```python
from build123d import *

# Parameters (mm, degrees)
SALIENTE_EXTRUIR1_DEPTH  = 2
CROQUIS2_W               = 30
CROQUIS2_H               = 17
CORTAR_EXTRUIR1_DEPTH    = 8
CROQUIS4_W               = 63.5
CROQUIS4_H               = 4
SALIENTE_EXTRUIR2_DEPTH  = 48.5
CROQUIS5_W               = 43.5
CROQUIS5_H               = 2.5
SALIENTE_EXTRUIR3_DEPTH  = 35
CROQUIS7_R               = 1.5
CORTAR_EXTRUIR2_DEPTH    = 9
CROQUIS8_R               = 1.5
CORTAR_EXTRUIR3_DEPTH    = 23
SALIENTE_EXTRUIR4_DEPTH  = 2
CROQUIS13_R              = 1.5
CORTAR_EXTRUIR4_DEPTH    = 2
CROQUIS16_W              = 3
CROQUIS16_H              = 31
SALIENTE_EXTRUIR7_DEPTH  = 2
CROQUIS17_W              = 15
CROQUIS17_H              = 3
SALIENTE_EXTRUIR8_DEPTH  = 25
CROQUIS21_W              = 15
CROQUIS21_H              = 3
SALIENTE_EXTRUIR9_DEPTH  = 2
CROQUIS25_R              = 3.826074219
CORTAR_EXTRUIR6_DEPTH    = 2
CROQUIS28_W              = 44.201296129
CROQUIS28_H              = 11.418561917
SALIENTE_EXTRUIR10_DEPTH = 2
CROQUIS30_W              = 15
CROQUIS30_H              = 3
SALIENTE_EXTRUIR11_DEPTH = 8
CROQUIS31_W              = 14
CROQUIS31_H              = 9
CORTAR_EXTRUIR7_DEPTH    = 2
CROQUIS33_W              = 39.5
CROQUIS33_H              = 1
SALIENTE_EXTRUIR13_DEPTH = 2
CROQUIS36_W              = 4.944902354
CROQUIS36_H              = 4.974433571
CROQUIS36_R              = 1.566702584
SALIENTE_EXTRUIR14_DEPTH = 2
CROQUIS37_R              = 2.242266835
CORTAR_EXTRUIR8_DEPTH    = 2
CROQUIS38_W              = 1.939564783
CROQUIS38_H              = 6.647351579
SALIENTE_EXTRUIR18_DEPTH = 2
CROQUIS39_R              = 2.608387943
CORTAR_EXTRUIR9_DEPTH    = 2
CROQUIS40_R              = 2.045540146
CORTAR_EXTRUIR10_DEPTH   = 2
CROQUIS41_R              = 2.280483158
CORTAR_EXTRUIR11_DEPTH   = 2
CROQUIS42_W              = 15
CROQUIS42_H              = 25
SALIENTE_EXTRUIR19_DEPTH = 5
CROQUIS43_R              = 1.6
CORTAR_EXTRUIR12_DEPTH   = 10


with BuildPart() as part:
    # Croquis1 → Saliente-Extruir1 (new body)
    with BuildSketch(Plane(origin=(0, 0, 0), x_dir=(1, 0, 0), z_dir=(0, 1, 0))):
        Polygon((25, 42), (-25, 42), (-25, -29), (-50, -29), (-50, -42), (50, -42), (50, -29), (25, -29), align=None)
    extrude(amount=SALIENTE_EXTRUIR1_DEPTH)

    # Croquis2 → Cortar-Extruir1 (cut)
    with BuildSketch(Plane(origin=(0, 0, 0), x_dir=(1, 0, 0), z_dir=(0, 1, 0))):
        with Locations((0, 33.5)):
            Rectangle(CROQUIS2_W, CROQUIS2_H)
    extrude(amount=CORTAR_EXTRUIR1_DEPTH, mode=Mode.SUBTRACT)

    # Croquis4 → Saliente-Extruir2 (add)
    with BuildSketch(Plane(origin=(0, 0, 0), x_dir=(1, 0, 0), z_dir=(0, 1, 0))):
        with Locations((0, -40)):
            Rectangle(CROQUIS4_W, CROQUIS4_H)
    extrude(amount=SALIENTE_EXTRUIR2_DEPTH)

    # Croquis5 → Saliente-Extruir3 (add)
    with BuildSketch(Plane(origin=(0, 0, 0), x_dir=(1, 0, 0), z_dir=(0, 1, 0))):
        with Locations((0, -3.75)):
            Rectangle(CROQUIS5_W, CROQUIS5_H)
    extrude(amount=SALIENTE_EXTRUIR3_DEPTH)

    # Croquis7 → Cortar-Extruir2 (cut, symmetric)
    with BuildSketch(Plane(origin=(0, 0, 38), x_dir=(-1, 0, 0), z_dir=(0, 0, -1))):
        with Locations(Location((-18, 43.25, 0), (0, 0, 180))):
            Circle(CROQUIS7_R)
        with Locations(Location((18, 43.25, 0), (0, 0, 180))):
            Circle(CROQUIS7_R)
        with Locations(Location((18, 7.25, 0), (0, 0, 180))):
            Circle(CROQUIS7_R)
        with Locations(Location((-18, 7.25, 0), (0, 0, 180))):
            Circle(CROQUIS7_R)
    extrude(amount=CORTAR_EXTRUIR2_DEPTH, both=True, mode=Mode.SUBTRACT)

    # Croquis8 → Cortar-Extruir3 (cut)
    with BuildSketch(Plane(origin=(0, 0, 2.5), x_dir=(-1, 0, 0), z_dir=(0, 0, -1))):
        with Locations((-15, 27.5)):
            Circle(CROQUIS8_R)
        with Locations((15, 9.5)):
            Circle(CROQUIS8_R)
        with Locations((15, 27.5)):
            Circle(CROQUIS8_R)
        with Locations((-15, 9.5)):
            Circle(CROQUIS8_R)
    extrude(amount=-CORTAR_EXTRUIR3_DEPTH, mode=Mode.SUBTRACT)



with BuildPart() as body_2:
    # Croquis12 → Saliente-Extruir4 (new body)
    with BuildSketch(Plane(origin=(0, 35, -35), x_dir=(1, 0, 0), z_dir=(0, -1, 0))):
        Polygon((21.25, 44.75), (-21.25, 44.75), (-21.25, 54.25), (-30.25, 54.25), (-30.25, 23.25), (-21.25, 23.25), (-21.25, 32.75), (21.25, 32.75), (21.25, 23.25), (30.25, 23.25), (30.25, 54.25), (21.25, 54.25), align=None)
    extrude(amount=-SALIENTE_EXTRUIR4_DEPTH)

    # Croquis13 → Cortar-Extruir4 (cut)
    with BuildSketch(Plane(origin=(0, 37, 0), x_dir=(1, 0, 0), z_dir=(0, 1, 0))):
        with Locations(Location((23, -15.25, 0), (0, 0, 270))):
            Circle(CROQUIS13_R)
        with Locations(Location((23, 7.75, 0), (0, 0, 90))):
            Circle(CROQUIS13_R)
        with Locations(Location((-23, 7.75, 0), (0, 0, 270))):
            Circle(CROQUIS13_R)
        with Locations(Location((-23, -15.25, 0), (0, 0, 90))):
            Circle(CROQUIS13_R)
    extrude(amount=-CORTAR_EXTRUIR4_DEPTH, mode=Mode.SUBTRACT)


with BuildPart() as part_1:
    add(part.part)

    add(body_2.part)  # Saliente-Extruir7 merges body 2
    # Croquis16 → Saliente-Extruir7 (add)
    with BuildSketch(Plane(origin=(0, 37, 0), x_dir=(1, 0, 0), z_dir=(0, 1, 0))):
        with Locations((-19.75, -3.75)):
            Rectangle(CROQUIS16_W, CROQUIS16_H)
    extrude(amount=-SALIENTE_EXTRUIR7_DEPTH)

    # Croquis17 → Saliente-Extruir8 (add)
    with BuildSketch(Plane(origin=(0, 2, 0), x_dir=(1, 0, 0), z_dir=(0, 1, 0))):
        with Locations((-0.769919921, 23.5)):
            Rectangle(CROQUIS17_W, CROQUIS17_H)
    extrude(amount=SALIENTE_EXTRUIR8_DEPTH)

    # Croquis21 → Saliente-Extruir9 (add)
    with BuildSketch(Plane(origin=(0, 27, 0), x_dir=(1, 0, 0), z_dir=(0, 1, 0))):
        with Locations((-0.769919921, 23.5)):
            Rectangle(CROQUIS21_W, CROQUIS21_H)
    extrude(amount=SALIENTE_EXTRUIR9_DEPTH)

    # Croquis25 → Cortar-Extruir6 (cut)
    with BuildSketch(Plane(origin=(0, 0, -25), x_dir=(-1, 0, 0), z_dir=(0, 0, -1))):
        with Locations((1.065680286, 20.360266958)):
            Circle(CROQUIS25_R)
    extrude(amount=-CORTAR_EXTRUIR6_DEPTH, mode=Mode.SUBTRACT)

    # Croquis28 → Saliente-Extruir10 (add)
    with BuildSketch(Plane(origin=(0, 37, 0), x_dir=(1, 0, 0), z_dir=(0, 1, 0))):
        with Locations((0.855508958, 17.459280959)):
            Rectangle(CROQUIS28_W, CROQUIS28_H)
    extrude(amount=-SALIENTE_EXTRUIR10_DEPTH)

    # Croquis30 → Saliente-Extruir11 (add)
    with BuildSketch(Plane(origin=(0, 37, 0), x_dir=(1, 0, 0), z_dir=(0, 1, 0))):
        with Locations((-0.769919921, 23.5)):
            Rectangle(CROQUIS30_W, CROQUIS30_H)
    extrude(amount=-SALIENTE_EXTRUIR11_DEPTH)

    # Croquis31 → Cortar-Extruir7 (cut)
    with BuildSketch(Plane(origin=(0, 37, 0), x_dir=(1, 0, 0), z_dir=(0, 1, 0))):
        with Locations((-1.129241311, 17.391372283)):
            Rectangle(CROQUIS31_W, CROQUIS31_H)
    extrude(amount=-CORTAR_EXTRUIR7_DEPTH, mode=Mode.SUBTRACT)

    # Croquis33 → Saliente-Extruir13 (add)
    with BuildSketch(Plane(origin=(0, 37, 0), x_dir=(1, 0, 0), z_dir=(0, 1, 0))):
        with Locations((1.5, 11.25)):
            Rectangle(CROQUIS33_W, CROQUIS33_H)
    extrude(amount=-SALIENTE_EXTRUIR13_DEPTH)

    # Croquis36 → Saliente-Extruir14 (add)
    with BuildSketch(Plane(origin=(0, 37, 0), x_dir=(1, 0, 0), z_dir=(0, 1, 0))):
        with Locations((23.722451177, 7.461073997)):
            Rectangle(CROQUIS36_W, CROQUIS36_H)
        with Locations((23.477387718, 7.75)):
            Circle(CROQUIS36_R, mode=Mode.SUBTRACT)
    extrude(amount=-SALIENTE_EXTRUIR14_DEPTH)

    # Croquis37 → Cortar-Extruir8 (cut)
    with BuildSketch(Plane(origin=(0, 37, 0), x_dir=(1, 0, 0), z_dir=(0, 1, 0))):
        with Locations((24.186288099, 7.75)):
            Circle(CROQUIS37_R)
    extrude(amount=-CORTAR_EXTRUIR8_DEPTH, mode=Mode.SUBTRACT)

    # Croquis38 → Saliente-Extruir18 (add)
    with BuildSketch(Plane(origin=(0, 37, 0), x_dir=(1, 0, 0), z_dir=(0, 1, 0))):
        with Locations((22.219782392, -15.926324211)):
            Rectangle(CROQUIS38_W, CROQUIS38_H)
    extrude(amount=-SALIENTE_EXTRUIR18_DEPTH)

    # Croquis39 → Cortar-Extruir9 (cut)
    with BuildSketch(Plane(origin=(0, 37, 0), x_dir=(1, 0, 0), z_dir=(0, 1, 0))):
        with Locations(Location((24.5, -15.25, 0), (0, 0, 270))):
            Circle(CROQUIS39_R)
    extrude(amount=-CORTAR_EXTRUIR9_DEPTH, mode=Mode.SUBTRACT)

    # Croquis40 → Cortar-Extruir10 (cut)
    with BuildSketch(Plane(origin=(0, 37, 0), x_dir=(1, 0, 0), z_dir=(0, 1, 0))):
        with Locations(Location((-23, 7.75, 0), (0, 0, 270))):
            Circle(CROQUIS40_R)
    extrude(amount=-CORTAR_EXTRUIR10_DEPTH, mode=Mode.SUBTRACT)

    # Croquis41 → Cortar-Extruir11 (cut)
    with BuildSketch(Plane(origin=(0, 37, 0), x_dir=(1, 0, 0), z_dir=(0, 1, 0))):
        with Locations(Location((-23, -15.25, 0), (0, 0, 270))):
            Circle(CROQUIS41_R)
    extrude(amount=-CORTAR_EXTRUIR11_DEPTH, mode=Mode.SUBTRACT)

    # Croquis42 → Saliente-Extruir19 (add)
    with BuildSketch(Plane(origin=(0, 0, -25), x_dir=(-1, 0, 0), z_dir=(0, 0, -1))):
        with Locations((0.769919921, 14.5)):
            Rectangle(CROQUIS42_W, CROQUIS42_H)
    extrude(amount=-SALIENTE_EXTRUIR19_DEPTH)

    # Croquis43 → Cortar-Extruir12 (cut)
    with BuildSketch(Plane(origin=(0, 2, 0), x_dir=(1, 0, 0), z_dir=(0, 1, 0))):
        with Locations(Location((-20, 38, 0), (0, 0, 270))):
            Circle(CROQUIS43_R)
        with Locations(Location((20, 38, 0), (0, 0, 270))):
            Circle(CROQUIS43_R)
        with Locations(Location((-35, -35, 0), (0, 0, 270))):
            Circle(CROQUIS43_R)
        with Locations(Location((35, -35, 0), (0, 0, 270))):
            Circle(CROQUIS43_R)
    extrude(amount=-CORTAR_EXTRUIR12_DEPTH, mode=Mode.SUBTRACT)


solid = part_1.part
```
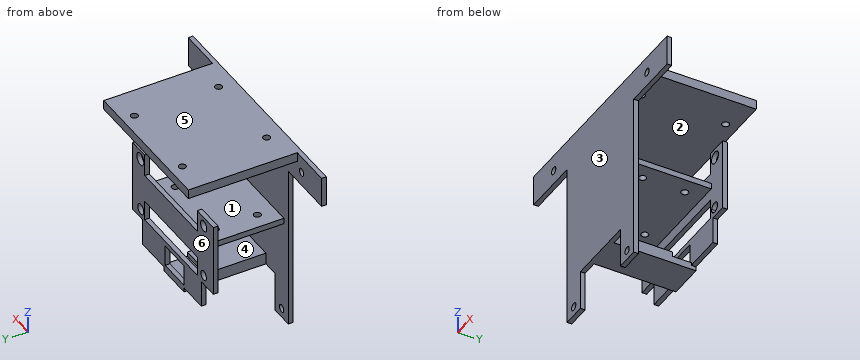
Here's how the part is built. I have some questions about the finished solid (model axes, mm). Face numbers are marked on the shaded views. A direction names the side the tool comes from. Coordinates: 2 decimals unless noted, no trailing zeros. Order: outer loops, then holes, each group sorted by start corner. A loop starts at its lowest first (then second) coordinate and runs counter-clockwise, first axis right, second up.
1) I need wall thicknesses on line 1 (Y direction, x = -18, z = 40); line 2 (X direction, y = 7.25, z = 40.7); line 3 (Y direction, x = -15, z = 3). Which ranges of each line are inside material? Lowest first, please.
2) Imagine slicing it at D-D on z = 31.5. List the corners of the cut face in (x, y) for me.
3) Imagine slicing it at B-B on z = 11.5. List the corners of the cut face in (x, y) for me, and give its area (3 significant figures).
4) We'd pull the mould along Z, two halves only. Please class the marked faces 4, 5 and 6: +Z half, -Z half, draft (parallel to the pull), parting line (faces both ways), or undercut.
5) Will these pins go through, and if not, where does the flat tip stop? pin 1 (4 mm diameter, centred on x = 3.5, z = 7, fed in from +Y); pin 2 (14 mm diameter, centred on x = 11, y = 35.5, fed in from -Z); pin 3 (0.6 mm diameter, centred on y = 1, z = -9.5, fed in from -X).
6) Imagine slicing it at C-C on z = -34. List the corners of the cut face in (x, y) for me, and give its area (3 significant figures).
7) Imagine slicing it at A-A on z = 0. List the corners of the cut face in (x, y) for me.
8) Which directions (+Z, -Z, +X, -X, +Y, -Y) give clear straight access to the entire face, cutting with the end or side of a thin tool? Please do the marked faces 1, 2 and 3.
Response values:
1. line 1: y = 0 to 5.75, 8.75 to 41.75, 44.75 to 48.5
1. line 2: x = -31.75 to -19.5, -16.5 to 16.5, 19.5 to 31.75
1. line 3: y = 0 to 8, 11 to 26, 29 to 37
2. outline: (-50, 0) - (50, 0) - (50, 2) - (-50, 2) - close
3. outline: (-30.25, 35) - (-18.25, 35) - (-18.25, 37) - (-30.25, 37) - close; (-25, 0) - (25, 0) - (25, 2) - (-25, 2) - close; (21.25, 35) - (30.25, 35) - (30.25, 37) - (21.25, 37) - close
3. area: 142 mm2
4. face 4: undercut
4. face 5: +Z half
4. face 6: draft
5. pin 1: stops at y = 37
5. pin 2: stops at z = -25
5. pin 3: stops at x = -25
6. outline: (-25, 0) - (-15, 0) - (-15, 2) - (-25, 2) - close; (15, 0) - (25, 0) - (25, 2) - (15, 2) - close
6. area: 40.0 mm2
7. outline: (-30.25, 35) - (30.25, 35) - (30.25, 37) - (-30.25, 37) - close; (-25, 0) - (25, 0) - (25, 2) - (-25, 2) - close
8. face 1: +X, -X
8. face 2: +X, -X, +Y
8. face 3: +Z, -Z, +X, -X, -Y
